from build123d import *

# Parameters (mm, degrees)
BOSS_EXTRUDE1_DEPTH      = 6.35
BOSS_EXTRUDE1_DEPTH_BACK = 6.35
SKETCH2_R                = 1.733880633
FILLET1_R                = 10.16
BOSS_EXTRUDE3_DEPTH      = 3.175
SKETCH7_R                = 1.7526
CUT_EXTRUDE3_DEPTH       = 22.606


with BuildPart() as part:
    # Sketch2 → Boss-Extrude1 (new, two sides: drawn at the far end of the back side and taken through both)
    with BuildSketch(Plane(origin=(0, 13820.707967808, 11763.157588594), x_dir=(0, 0.8457184946773667, 0.533629298071844), z_dir=(1, 0, 0)).offset(-BOSS_EXTRUDE1_DEPTH_BACK)):
        with BuildLine():
            Line((77.82010292, 2.698073613), (77.82010292, -12.045648124))
            ThreePointArc((77.82010292, -12.045648124), (78.936026083, -14.73972496), (81.63010292, -15.855648124))
            Line((81.63010292, -15.855648124), (84.011557282, -15.855648124))
            ThreePointArc((84.011557282, -15.855648124), (86.705634118, -14.73972496), (87.821557282, -12.045648124))
            Line((87.821557282, -12.045648124), (87.821557282, 2.698073613))
            Line((87.821557282, 2.698073613), (87.821557282, 9.367220025))
            ThreePointArc((87.821557282, 9.367220025), (89.681429221, 13.857348086), (94.171557282, 15.717220025))
            Line((94.171557282, 15.717220025), (104.328561269, 15.717220025))
            Line((104.328561269, 15.717220025), (104.328561269, 25.877220025))
            Line((104.328561269, 25.877220025), (59.175813007, 25.877220025))
            ThreePointArc((59.175813007, 25.877220025), (56.544296522, 25.306287509), (54.385982659, 23.696155769))
            Line((54.385982659, 23.696155769), (44.81523307, 12.7))
            Line((44.81523307, 12.7), (53.583504994, 12.7))
            Line((53.583504994, 12.7), (54.97523307, 12.7))
            Line((54.97523307, 12.7), (56.039282698, 13.597053748))
            Line((56.039282698, 13.597053748), (58.554139967, 15.717220025))
            Line((58.554139967, 15.717220025), (71.47010292, 15.717220025))
            ThreePointArc((71.47010292, 15.717220025), (75.96023098, 13.857348086), (77.82010292, 9.367220025))
            Line((77.82010292, 9.367220025), (77.82010292, 2.698073613))
        make_face()
        with Locations(Location((82.820830101, -2.442575088, 0), (0, 0, 237.748998542))):
            Circle(SKETCH2_R, mode=Mode.SUBTRACT)
    extrude(amount=BOSS_EXTRUDE1_DEPTH + BOSS_EXTRUDE1_DEPTH_BACK)

    # Fillet1
    fillet1_edges = [part.edges().sort_by_distance(p)[0] for p in [
        (0, 13895.131718838, 11840.715209079),
    ]]
    fillet(fillet1_edges, radius=FILLET1_R - 0.0001)  # a hair under: the kernel refuses the full size

    # Sketch5 → Boss-Extrude3 (add)
    with BuildSketch(Plane(origin=(0, -1379.90412378, 2186.930969826), x_dir=(-1, 0, 0), z_dir=(0, 0.5336292980726433, -0.8457184946768624))):
        Polygon((4.826, 18020.569098092), (4.826, 18011.9803546), (4.826, 18010.409098092), (6.35, 18010.409098092), (6.35, 18012.025656104), (6.35, 18020.569098092), align=None)
        Polygon((-6.35, 18011.9803546), (-6.35, 18020.569098092), (-4.826, 18020.569098092), (-4.826, 18011.9803546), (-4.826, 18010.409098092), (-6.35, 18010.409098092), align=None)
    extrude(amount=BOSS_EXTRUDE3_DEPTH)

    # Sketch7 → Cut-Extrude3 (cut)
    with BuildSketch(Plane(origin=(6.35, 0, 0), x_dir=(0, 0, -1), z_dir=(1, 0, 0))):
        with Locations((-11832.634859183, 13894.225281819)):
            Circle(SKETCH7_R)
    extrude(amount=-CUT_EXTRUDE3_DEPTH, mode=Mode.SUBTRACT)


solid = part.part
Could you check a few things on this model? Use its own coordinates, in mm. A direction names the side the tool comes from. Give positions to 0.01 mm unless a question says otherwise; leave off trailing zeros. Order: outer loops, then holes, each group sorted by start corner. A loop starts at its lowest first (then second) coordinate and runs counter-clockwise, first axis right, second up.
1. Suppose I cut it at A-A (z = 11833.5). List the corners of the cut face in (x, y) for me.
2. Will these pins go through, and if not, where does the flat tip stop? P1, Ø2, axis at x = 4, z = 11824, coming from the -Y side; P2, Ø1, axis at x = -4, y = 13867.5, coming from the -Z side; P3, Ø4, axis at x = -0.5, z = 11819.5, coming from the +Y side; P4, Ø2, axis at y = 13867, z = 11807.5, coming from the -X side.
3. Suppose I cut it at B-B (y = 13897.5). List the corners of the cut face in (x, z) for me, plus the area to 3 significant figures.
4. Suppose I cut it at C-C (z = 11806). List the corners of the cut face in (x, y) for me, plus the area to 3 significant figures.
5. Suppose I cut it at D-D (x = -4). Give the number of separate pieces and of enclosed holes in the cut face, plus the area to 3 significant figures.
6. For faces 5 (the flat face through (-0.089, 13896.198, 11829.375)), 6 (the flat face through (-5.6, 13861.26, 11801.91)), 7 (the flat face through (-0.068, 13856.068, 11800.486)), 8 (the flat face through (5.577, 13857.883, 11797.877)), which set-ups out of +Z, -Z, +X, -X, +Y, -Y let a thin tool reach every point of the face, with its end or its side?
7. I need wall thicknesses on L1, parallel to Z at x = 3.75, y = 13894.5; L2, parallel to Z at x = -5.75, y = 13893.5; L3, parallel to Y at x = -3, z = 11834. Which ranges of each line are inside material? Lowest first, please.
8. We'd pull the mould along Y, two halves only. Please class faces 1 (the flat face through (-0.089, 13895.775, 11808.762)), 2 (the flat face through (-6.35, 13884, 11815)), 3 (the flat face through (-0.089, 13887.157, 11803.679)), 4 (the flat face through (-4.826, 13857, 11799)): pulls with the +Y half, pulls with the -Y half, needs draft (parallel to the pull), parting line crosses it, or undercut.
Solved:
1. outline: (-6.35, 13883.7) - (6.35, 13883.7) - (6.35, 13892.7) - (-6.35, 13892.7) - close; (-6.35, 13895.75) - (6.35, 13895.75) - (6.35, 13899.51) - (-6.35, 13899.51) - close
2. P1: stops at y = 13867.06
2. P2: stops at z = 11810.95
2. P3: stops at y = 13890.26
2. P4: passes through
3. outline: (-6.35, 11792.96) - (6.35, 11792.96) - (6.35, 11806.03) - (-6.35, 11806.03) - close; (-6.35, 11830.2) - (6.35, 11830.2) - (6.35, 11835.22) - (-6.35, 11835.22) - close
3. area: 230 mm2
4. outline: (-6.35, 13853.1) - (6.35, 13853.1) - (6.35, 13861.3) - (-6.35, 13861.3) - close; (-6.35, 13885.69) - (6.35, 13885.69) - (6.35, 13890.47) - (-6.35, 13890.47) - close; (-6.35, 13893.64) - (6.35, 13893.64) - (6.35, 13897.52) - (-6.35, 13897.52) - close
4. area: 214 mm2
5. separate pieces: 1
5. enclosed holes: 2
5. area: 850 mm2
6. face 5: +X, -X, +Y
6. face 6: +X, -X
6. face 7: -Z
6. face 8: -Z, +X, -X
7. L1: z = 11793.11 to 11810.78, 11828.3 to 11830.9, 11834.37 to 11836.54
7. L2: z = 11793.81 to 11804.33, 11806.25 to 11812.37, 11827.67 to 11831.04, 11834.23 to 11836.74
7. L3: y = 13884.49 to 13893.13, 13895.32 to 13899.03
8. face 1: pulls with the +Y half
8. face 2: needs draft
8. face 3: undercut
8. face 4: undercut
